from build123d import *

# Parameters (mm, degrees)
SKETCH1_W           = 355.6
SKETCH1_H           = 609.6
SKETCH1_W_2         = 304.8
SKETCH1_H_2         = 558.8
BOSS_EXTRUDE2_DEPTH = 203.2
SKETCH4_W           = 304.8
SKETCH4_H           = 558.8
BOSS_EXTRUDE3_DEPTH = 50.8
SKETCH5_R           = 6.35
CUT_EXTRUDE1_DEPTH  = 25.4
SKETCH6_R           = 6.35
CUT_EXTRUDE2_DEPTH  = 12.7


with BuildPart() as part:
    # Sketch1 → Boss-Extrude2 (new body)
    with BuildSketch(Plane.XY):
        with Locations((177.8, 304.8)):
            Rectangle(SKETCH1_W, SKETCH1_H)
        with Locations((177.8, 304.8)):
            Rectangle(SKETCH1_W_2, SKETCH1_H_2, mode=Mode.SUBTRACT)
    extrude(amount=BOSS_EXTRUDE2_DEPTH)

    # Sketch4 → Boss-Extrude3 (add)
    with BuildSketch(Plane(origin=(0, 0, 0), x_dir=(-1, 0, 0), z_dir=(0, 0, -1))):
        with Locations((-177.8, 304.8)):
            Rectangle(SKETCH4_W, SKETCH4_H)
    extrude(amount=-BOSS_EXTRUDE3_DEPTH)

    # Sketch5 → Cut-Extrude1 (cut)
    with BuildSketch(Plane.XY.offset(203.2)):
        with Locations((11.88567414, 50.947353246)):
            Circle(SKETCH5_R)
        with Locations((11.88567414, 101.747353246)):
            Circle(SKETCH5_R)
        with Locations((11.88567414, 507.852646754)):
            Circle(SKETCH5_R)
        with Locations((11.88567414, 558.652646754)):
            Circle(SKETCH5_R)
        with Locations((343.71432586, 50.947353246)):
            Circle(SKETCH5_R)
        with Locations((343.71432586, 101.747353246)):
            Circle(SKETCH5_R)
        with Locations((343.71432586, 558.652646754)):
            Circle(SKETCH5_R)
        with Locations((343.71432586, 507.852646754)):
            Circle(SKETCH5_R)
    extrude(amount=-CUT_EXTRUDE1_DEPTH, mode=Mode.SUBTRACT)

    # Sketch6 → Cut-Extrude2 (cut)
    with BuildSketch(Plane.XY.offset(203.2)):
        with Locations((343.71432586, 596.9)):
            Circle(SKETCH6_R)
        with Locations((177.8, 596.9)):
            Circle(SKETCH6_R)
        with Locations((11.88567414, 596.9)):
            Circle(SKETCH6_R)
        with Locations((343.71432586, 12.7)):
            Circle(SKETCH6_R)
        with Locations((177.8, 12.7)):
            Circle(SKETCH6_R)
        with Locations((11.88567414, 12.7)):
            Circle(SKETCH6_R)
    extrude(amount=-CUT_EXTRUDE2_DEPTH, mode=Mode.SUBTRACT)


solid = part.part
Geometry: final body of the model. Coordinates: model frame, mm. Round coordinates to 2 decimals unless told otherwise and drop trailing zeros. Loops run counter-clockwise (first coordinate to the right, second up) from the corner with the lowest first, then second, coordinate; pieces in that order, holes last.
Q1. Section B-B on x = 61. Return loops of the section in (y, z).
Q2. Pull-direction query (X, two-part tool) for faces 1 (the cylindrical face through (11.059, 57.243, 190.678)), 2 (the flat face through (19, 284, 203.2)), 3 (the flat face through (344, 51, 177.8)), 4 (the flat face through (0, 301, 100)); classes: released by +X, released by -X, zero draft, split by the parting line, or undercut.
Q3. Section C-C on y = 360.5. Return loops of the section in (x, z), plus the area to 3 significant figures.
Q4. Material intervals for L1, parallel to X at y = 12, z = 199; L2, parallel to X at y = 596.9, z = 196; L3, parallel to X at y = 479, z = 162, sorted ascending.
Q5. Pin query (flat end, axial travel): P1, Ø4, axis at x = 13.5, y = 594, coming from the +Z side; P2, Ø11.5, axis at x = 11.89, y = 101.75, coming from the +Z side. Return the tip coordinate at first contact, or that it passes through.
Q6. Section D-D on x = 177.8. Return loops of the section in (y, z).
Q7. Section A-A on z = 73. Return loops of the section in (x, y).
Evaluation:
1. outline: (0, 0) - (609.6, 0) - (609.6, 203.2) - (584.2, 203.2) - (584.2, 50.8) - (25.4, 50.8) - (25.4, 203.2) - (0, 203.2) - close
2. face 1: undercut
2. face 2: zero draft
2. face 3: undercut
2. face 4: released by -X
3. outline: (0, 0) - (355.6, 0) - (355.6, 203.2) - (330.2, 203.2) - (330.2, 50.8) - (25.4, 50.8) - (25.4, 203.2) - (0, 203.2) - close
3. area: 25,800 mm2
4. L1: x = 0 to 5.57, 18.2 to 171.49, 184.11 to 337.4, 350.03 to 355.6
4. L2: x = 0 to 5.54, 18.24 to 171.45, 184.15 to 337.36, 350.06 to 355.6
4. L3: x = 0 to 25.4, 330.2 to 355.6
5. P1: stops at z = 190.5
5. P2: stops at z = 177.8
6. outline: (0, 0) - (609.6, 0) - (609.6, 203.2) - (603.25, 203.2) - (603.25, 190.5) - (590.55, 190.5) - (590.55, 203.2) - (584.2, 203.2) - (584.2, 50.8) - (25.4, 50.8) - (25.4, 203.2) - (19.05, 203.2) - (19.05, 190.5) - (6.35, 190.5) - (6.35, 203.2) - (0, 203.2) - close
7. outline: (0, 0) - (355.6, 0) - (355.6, 609.6) - (0, 609.6) - close; hole (25.4, 25.4) - (330.2, 25.4) - (330.2, 584.2) - (25.4, 584.2) - close
